```python
from build123d import *

# Parameters (mm, degrees)
SKETCH2_W           = 12.7
SKETCH2_H           = 22.225
BOSS_EXTRUDE2_DEPTH = 4.2926
BOSS_EXTRUDE3_DEPTH = 4.2926
CUT_EXTRUDE1_DEPTH  = 4.2926
FILLET3_R           = 1.27
SKETCH5_W           = 4.2926
SKETCH5_H           = 31.75
CUT_EXTRUDE2_DEPTH  = 4.2926
SKETCH6_W           = 4.2926
SKETCH6_H           = 38.1
CUT_EXTRUDE3_DEPTH  = 4.2926
SKETCH9_W           = 4.2926
SKETCH9_H           = 44.45
BOSS_EXTRUDE4_DEPTH = 6.35
SKETCH10_W          = 4.2926
SKETCH10_H          = 6.35
BOSS_EXTRUDE5_DEPTH = 6.35
SKETCH12_W          = 4.2926
SKETCH12_H          = 44.45
BOSS_EXTRUDE6_DEPTH = 8.382
FILLET4_R           = 1.27


with BuildPart() as part:
    # Sketch2 → Boss-Extrude2 (new body)
    with BuildSketch(Plane.XY):
        Polygon((6.35, 22.225), (6.35, 101.6), (-6.35, 101.6), (-6.35, 49.06413634), (-6.35, 22.225), align=None)
        with Locations((0, 11.1125)):
            Rectangle(SKETCH2_W, SKETCH2_H)
        Polygon((10.541, 22.225), (6.35, 22.225), (6.35, 0), (-6.35, 0), (-6.35, 22.225), (-10.541, 22.225), (-10.541, -22.225), (10.541, -22.225), align=None)
    extrude(amount=BOSS_EXTRUDE2_DEPTH)

    # Sketch2_3 → Boss-Extrude3 (add)
    with BuildSketch(Plane.XY):
        Polygon((-6.35, 101.6), (6.35, 101.6), (6.35, 186.37430696), (-74.996081542, 49.06413634), (-6.35, 49.06413634), align=None)
    extrude(amount=BOSS_EXTRUDE3_DEPTH)

    # Sketch4 → Cut-Extrude1 (cut)
    with BuildSketch(Plane(origin=(0, 0, 0), x_dir=(-1, 0, 0), z_dir=(0, 0, -1))):
        Polygon((2.26175511, 137.499289153), (4.882176806, 110.262347972), (21.501956662, 111.86130989), align=None)
        Polygon((25.53449714, 98.932202401), (34.449187247, 60.416195476), (55.473168553, 54.188396298), align=None)
        Polygon((9.42992166, 86.270055499), (5.634016985, 54.421399088), (24.410527091, 58.107059129), align=None)
        Polygon((7.556063617, 101.433706887), (27.432097362, 64.067482354), (20.599137511, 101.433706887), align=None)
    extrude(amount=-CUT_EXTRUDE1_DEPTH, mode=Mode.SUBTRACT)

    # Fillet3
    fillet3_edges = [part.edges().sort_by_distance(p)[0] for p in [
        (6.35, 186.37430696, 2.1463),
        (-74.996081542, 49.06413634, 2.1463),
        (-6.35, 49.06413634, 2.1463),
        (-2.26175511, 137.499289153, 2.1463),
        (-21.501956662, 111.86130989, 2.1463),
        (-4.882176806, 110.262347972, 2.1463),
        (-20.599137511, 101.433706887, 2.1463),
        (-27.432097362, 64.067482354, 2.1463),
        (-7.556063617, 101.433706887, 2.1463),
        (-25.53449714, 98.932202401, 2.1463),
        (-55.473168553, 54.188396298, 2.1463),
        (-9.42992166, 86.270055499, 2.1463),
        (-24.410527091, 58.107059129, 2.1463),
        (-5.634016985, 54.421399088, 2.1463),
    ]]
    fillet(fillet3_edges, radius=FILLET3_R)

    # Sketch5 → Cut-Extrude2 (cut)
    with BuildSketch(Plane(origin=(0, 0, 0), x_dir=(-1, 0, 0), z_dir=(0, 0, -1))):
        with Locations((0, -6.35)):
            Rectangle(SKETCH5_W, SKETCH5_H)
    extrude(amount=-CUT_EXTRUDE2_DEPTH, mode=Mode.SUBTRACT)

    # Sketch6 → Cut-Extrude3 (cut)
    with BuildSketch(Plane(origin=(0, 0, 0), x_dir=(-1, 0, 0), z_dir=(0, 0, -1))):
        with Locations((-4.2926, -3.175)):
            Rectangle(SKETCH6_W, SKETCH6_H)
    extrude(amount=-CUT_EXTRUDE3_DEPTH, mode=Mode.SUBTRACT)

    # Sketch9 → Boss-Extrude4 (add)
    with BuildSketch(Plane(origin=(10.541, 0, 0), x_dir=(0, 0, -1), z_dir=(1, 0, 0))):
        with Locations((-2.1463, 0)):
            Rectangle(SKETCH9_W, SKETCH9_H)
    extrude(amount=BOSS_EXTRUDE4_DEPTH)

    # Sketch10 → Boss-Extrude5 (add)
    with BuildSketch(Plane(origin=(6.35, 0, 0), x_dir=(0, 0, -1), z_dir=(1, 0, 0))):
        with Locations((-2.1463, 25.4)):
            Rectangle(SKETCH10_W, SKETCH10_H)
    extrude(amount=BOSS_EXTRUDE5_DEPTH)

    # Sketch12 → Boss-Extrude6 (add)
    with BuildSketch(Plane.ZY.offset(10.541)):
        with Locations((2.1463, 0)):
            Rectangle(SKETCH12_W, SKETCH12_H)
    extrude(amount=BOSS_EXTRUDE6_DEPTH)

    # Fillet4
    fillet4_edges = [part.edges().sort_by_distance(p)[0] for p in [
        (-6.35, 22.225, 2.1463),
        (-2.1463, 9.525, 2.1463),
        (-2.1463, -22.225, 2.1463),
        (2.1463, 9.525, 2.1463),
        (2.1463, 15.875, 2.1463),
        (6.4389, -22.225, 2.1463),
        (6.4389, 15.875, 2.1463),
        (16.891, -22.225, 2.1463),
        (16.891, 22.225, 2.1463),
        (6.35, 28.575, 2.1463),
        (12.7, 28.575, 2.1463),
        (-18.923, -22.225, 2.1463),
        (-18.923, 22.225, 2.1463),
    ]]
    fillet(fillet4_edges, radius=FILLET4_R)


solid = part.part
```
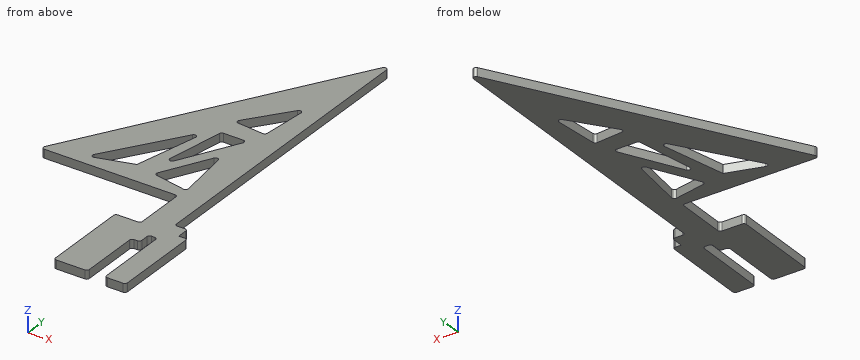
The listing builds one solid part. Answer for the finished solid, in the listing's coordinates (mm). Give positions to 0.01 mm unless a question says otherwise; leave off trailing zeros. Order: outer loops, then holes, each group sorted by start corner. A loop starts at its lowest first (then second) coordinate and runs counter-clockwise, first axis right, second up. Notation, with made-up numbers: (-1.5, 80) -> (26.5, 80) arc R19 cw to (26.5, 87) -> close; hole circle Ø9 at (42.5, 22.5). An arc over 180 degrees is marked (long way). Answer as a JSON object with one key per item and string values. Group by question number.
Item 1: The part is cut by section D-D on y = 169.5. Write down the section's boundary in (x, z).
Item 2: Consider L1, parallel to Y at x = -9.5, z = 0.95 (3 decimals); L2, parallel to X at y = -13, z = 3.35; L3, parallel to Y at x = -17.5, z = 3.3 (3 decimals). Determine where each line is inside the solid, lowest interval first. Write a range as from..to.
Item 3: Flat-ended cylindrical pins translate along their axes: pin 1 (2 mm diameter, centred on y = -3, z = 1.5, fed in from -X); pin 2 (1.3 mm diameter, centred on x = -47.5, z = 1.5, fed in from -Y); pin 3 (0.9 mm diameter, centred on x = 0, z = 3, fed in from -Y) (3 decimals). Find the tip coordinate at first contact, or state that the pin passes through.
Item 4: The part is cut by section B-B on x = -37.5. Write down the section's boundary in (y, z).
Item 5: The part is cut by section C-C on z = 1.15. Give the number of separate pieces and of enclosed holes in the cut face, and give its area (3 significant figures).
Item 6: The part is cut by section A-A on y = -7.5. Write down the section's boundary in (x, z), and give its area (3 significant figures).
Result set:
{
 "1": {"outline": "(-3.65, 0) -> (6.35, 0) -> (6.35, 4.29) -> (-3.65, 4.29) -> close"},
 "2": {"L1": "-22.225..22.225, 49.064..55.18, 83.148..97.779, 101.422..110.707, 127.854..159.62", "L2": "-18.92..-2.15, 6.44..16.89", "L3": "-22.225..22.225, 49.064..56.751, 71.099..82.739, 101.434..111.476, 117.194..146.116"},
 "3": {"pin 1": "x = -18.92", "pin 2": "y = 49.06", "pin 3": "y = 9.525"},
 "4": {"outline": "(49.06, 0) -> (59.51, 0) -> (59.51, 4.29) -> (49.06, 4.29) -> close; (81.05, 0) -> (112.36, 0) -> (112.36, 4.29) -> (81.05, 4.29) -> close"},
 "5": {"separate pieces": "1", "enclosed holes": "4", "area": "6,140 mm²"},
 "6": {"outline": "(-18.92, 0) -> (-2.15, 0) -> (-2.15, 4.29) -> (-18.92, 4.29) -> close; (6.44, 0) -> (16.89, 0) -> (16.89, 4.29) -> (6.44, 4.29) -> close", "area": "117 mm²"}
}
